```python
from build123d import *

# Parameters (mm, degrees)
F0_W     = 914.4
F0_H     = 609.6
F1_DEPTH = 19.05
F3_DEPTH = 25.4


with BuildPart() as f1:
    # F0 (on Top) → F1 (new body)
    with BuildSketch(Plane.XY):
        Rectangle(F0_W, F0_H)
    extrude(amount=F1_DEPTH)

    # F2 (on face) → F3 (cut)
    with BuildSketch(Plane.XY.offset(19.05)):
        with BuildLine():
            Line((0, 228.6), (12.7, 228.6))
            ThreePointArc((12.7, 228.6), (0, 241.3), (-12.7, 228.6))
            Line((-12.7, 228.6), (0, 228.6))
        make_face()
        with BuildLine():
            ThreePointArc((-12.7, 228.6), (0, 215.9), (12.7, 228.6))
            Line((12.7, 228.6), (0, 228.6))
            Line((0, 228.6), (-12.7, 228.6))
        make_face()
        with BuildLine():
            ThreePointArc((-12.7, -228.6), (0, -215.9), (12.7, -228.6))
            Line((12.7, -228.6), (12.7, 228.6))
            ThreePointArc((12.7, 228.6), (0, 215.9), (-12.7, 228.6))
            Line((-12.7, 228.6), (-12.7, -228.6))
        make_face()
        with BuildLine():
            Line((0, -228.6), (12.7, -228.6))
            ThreePointArc((12.7, -228.6), (0, -215.9), (-12.7, -228.6))
            Line((-12.7, -228.6), (0, -228.6))
        make_face()
        with BuildLine():
            ThreePointArc((-12.7, -228.6), (0, -241.3), (12.7, -228.6))
            Line((12.7, -228.6), (0, -228.6))
            Line((0, -228.6), (-12.7, -228.6))
        make_face()
    extrude(amount=-F3_DEPTH, mode=Mode.SUBTRACT)


solid = f1.part
```
The model under review builds one solid part; all positions refer to its coordinate system, in mm. A direction names the side the tool comes from. Round coordinates to 2 decimals unless told otherwise and drop trailing zeros. Order: outer loops, then holes, each group sorted by start corner. A loop starts at its lowest first (then second) coordinate and runs counter-clockwise, first axis right, second up. Notation, with made-up numbers: (18.5, -33) -> (26.5, -33) arc R22 ccw to (26.5, 4) -> close; hole circle Ø6 at (5, 14). An arc over 180 degrees is marked (long way). Use a Markdown table: item, result.
Q1. Tool access review of faces 4 (the flat face through (-6, -304.8, 9)), 5 (the cylindrical face through (-0.279, -241.297, 9.658)): name each direction out of +Z, -Z, +X, -X, +Y, -Y from which nothing blocks a thin tool from reaching the whole face with its end or side.
Values:
| item | result |
|---|---|
| face 4 | +Z, -Z, +X, -X, -Y |
| face 5 | +Z, -Z |
Q2. We need section A-A on y = -75.5. Write out the cut boundary in (x, z), then the cut area to 3 significant figures.
Values:
| item | result |
|---|---|
| outline | (-457.2, 0) -> (-12.7, 0) -> (-12.7, 19.05) -> (-457.2, 19.05) -> close; (12.7, 0) -> (457.2, 0) -> (457.2, 19.05) -> (12.7, 19.05) -> close |
| area | 16,900 mm^2 |
Q3. We need section C-C on z = 9.25. Write out the cut boundary in (x, y), then the cut area to 3 significant figures.
Values:
| item | result |
|---|---|
| outline | (-457.2, -304.8) -> (457.2, -304.8) -> (457.2, 304.8) -> (-457.2, 304.8) -> close; hole (-12.7, -228.6) arc R12.7 ccw to (12.7, -228.6) -> (12.7, 228.6) arc R12.7 ccw to (-12.7, 228.6) -> close |
| area | 545,000 mm^2 |
Q4. We need section B-B on x = 0. Write out the cut boundary in (y, z).
Values:
| item | result |
|---|---|
| outline | (-304.8, 0) -> (-241.3, 0) -> (-241.3, 19.05) -> (-304.8, 19.05) -> close; (241.3, 0) -> (304.8, 0) -> (304.8, 19.05) -> (241.3, 19.05) -> close |
Q5. For line 1 (X direction, y = 176, z = 4); line 2 (Y direction, x = 10, z = 4.25), list the stretches that pass through material, from the lowest coordinate up.
Values:
| item | result |
|---|---|
| line 1 | x = -457.2 to -12.7, 12.7 to 457.2 |
| line 2 | y = -304.8 to -236.43, 236.43 to 304.8 |
Q6. Mouldability with a two-part tool opening along Y and no side actions: class faces 1 (the cylindrical face through (0.279, 241.297, 9.658)), 2 (the flat face through (-6, 304.8, 9)), 3 (the flat face through (457.2, -4, 9)) as +Y half, -Y half, draft (parallel to the pull), parting line (faces both ways), or undercut.
Values:
| item | result |
|---|---|
| face 1 | undercut |
| face 2 | +Y half |
| face 3 | draft |
